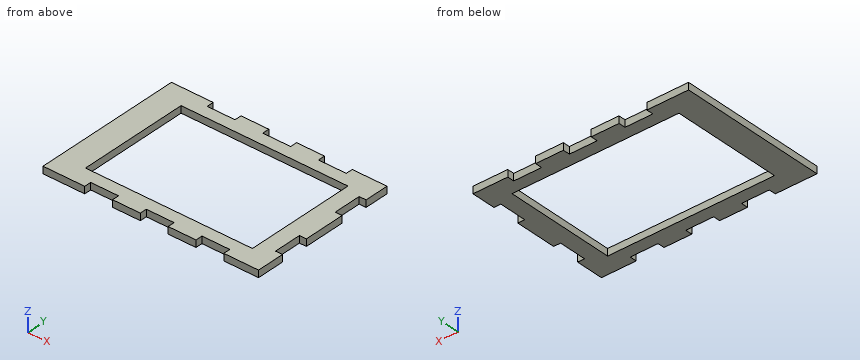
```python
from build123d import *

# Parameters (mm, degrees)
SKETCH1_W           = 196.85
SKETCH1_H           = 136.525
BOSS_EXTRUDE1_DEPTH = 6.35
SKETCH2_W           = 152.4
SKETCH2_H           = 101.6
CUT_EXTRUDE1_DEPTH  = 196.541125609
SKETCH3_W           = 6.35
SKETCH3_H           = 25.4
SKETCH3_H_2         = 25.381347512
SKETCH3_W_2         = 25.4
SKETCH3_H_3         = 6.35
CUT_EXTRUDE2_DEPTH  = 6.35


with BuildPart() as part:
    # Sketch1 → Boss-Extrude1 (new body)
    with BuildSketch(Plane.XY):
        with Locations((-33.205526088, -76.2)):
            Rectangle(SKETCH1_W, SKETCH1_H)
    extrude(amount=BOSS_EXTRUDE1_DEPTH)

    # Sketch2 → Cut-Extrude1 (cut, through all)
    with BuildSketch(Plane.XY.offset(6.35)):
        with Locations((-31.618026088, -76.2)):
            Rectangle(SKETCH2_W, SKETCH2_H)
    extrude(amount=-CUT_EXTRUDE1_DEPTH, mode=Mode.SUBTRACT)

    # Sketch3 → Cut-Extrude2 (cut)
    with BuildSketch(Plane(origin=(0, 0, 0), x_dir=(-1, 0, 0), z_dir=(0, 0, -1))):
        with Locations((-62.044473912, -106.3625)):
            Rectangle(SKETCH3_W, SKETCH3_H)
        with Locations((-62.044473912, -42.853173756)):
            Rectangle(SKETCH3_W, SKETCH3_H_2)
        with Locations((-20.769473912, -11.1125)):
            Rectangle(SKETCH3_W_2, SKETCH3_H_3)
        with Locations((30.030526088, -11.1125)):
            Rectangle(SKETCH3_W_2, SKETCH3_H_3)
        with Locations((80.830526088, -11.1125)):
            Rectangle(SKETCH3_W_2, SKETCH3_H_3)
        with Locations((-20.769473912, -141.2875)):
            Rectangle(SKETCH3_W_2, SKETCH3_H_3)
        with Locations((30.030526088, -141.2875)):
            Rectangle(SKETCH3_W_2, SKETCH3_H_3)
        with Locations((80.830526088, -141.2875)):
            Rectangle(SKETCH3_W_2, SKETCH3_H_3)
    extrude(amount=-CUT_EXTRUDE2_DEPTH, mode=Mode.SUBTRACT)


solid = part.part
```
The model under review builds one solid part; all positions refer to its coordinate system, in mm. Coordinates: 2 decimals unless noted, no trailing zeros. Write each loop counter-clockwise with the first axis right and the second up, starting at its lowest first coordinate (ties: lowest second). Pieces come first, ordered by that corner, then holes. Notation, with made-up numbers: (-13, -10) - (32, -10) arc R21 cw to (32, -4) - close; hole circle Ø8 at (-39.5, 62). An arc over 180 degrees is marked (long way). Write item = value, one per line.
(1) For P1, Ø1.9, axis at x = -28.5, z = 2, coming from the +Y side; P2, Ø1.5, axis at x = -84, z = 4.5, coming from the -Y side; P3, Ø1.9, axis at y = -105, z = 3, coming from the +X side, all flat-tipped, find the tip position at first contact; note any pin that passes through.
Result sheet:
P1 = -14.29
P2 = -138.11
P3 = 58.87
(2) For line 1 (Y direction, x = -78, z = 6); line 2 (X direction, y = -94.5, z = 6); line 3 (Y direction, x = 1, z = 3), list the stretches that pass through material, from the lowest coordinate up. Write a range as [from, to].
Result sheet:
line_1 = [-138.11, -127], [-25.4, -14.29]
line_2 = [-131.63, -107.82], [44.58, 58.87]
line_3 = [-144.46, -127], [-25.4, -7.94]
(3) Consider section A-A, the plane y = -35. Give the boundary of the cut face in (x, z), then the cut area to 3 significant figures.
Result sheet:
outline = (-131.63, 0) - (-107.82, 0) - (-107.82, 6.35) - (-131.63, 6.35) - close; (44.58, 0) - (58.87, 0) - (58.87, 6.35) - (44.58, 6.35) - close
area = 242 mm^2
(4) Consider section B-B, the plane x = -103.5. Give the boundary of the cut face in (y, z), then the cut area to 3 significant figures.
Result sheet:
outline = (-144.46, 0) - (-127, 0) - (-127, 6.35) - (-144.46, 6.35) - close; (-25.4, 0) - (-7.94, 0) - (-7.94, 6.35) - (-25.4, 6.35) - close
area = 222 mm^2
